Check sheet for the modelled part. Datum: model origin and axes. Units: mm. Give positions to 0.01 mm unless a question says otherwise; leave off trailing zeros. Write each loop counter-clockwise with the first axis right and the second up, starting at its lowest first coordinate (ties: lowest second). Pieces come first, ordered by that corner, then holes. Notation, with made-up numbers: (48, 28.5) -> (101, 28.5) arc R21 cw to (101, 53.5) -> close; hole circle Ø2 at (1, -27). An arc over 180 degrees is marked (long way). Answer as a JSON object with one key per item and string values.
from build123d import *

# Parameters (mm, degrees)
F1_DEPTH = 0.8128
F2_R     = 4.5
F3_DEPTH = 25.4


with BuildPart() as f1:
    # F0 (on Front) → F1 (new body)
    with BuildSketch(Plane.XZ):
        with BuildLine():
            ThreePointArc((-20.832611, 3.624153), (0, 21.1455), (20.832611, 3.624153))
            ThreePointArc((20.832611, 3.624153), (23.001379, -0.147215), (27.08865, -1.637512))
            Line((27.08865, -1.637512), (38.1, -1.637512))
            Line((38.1, -1.637512), (38.1, 33.287488))
            ThreePointArc((38.1, 33.287488), (36.240128, 37.777616), (31.75, 39.637488))
            Line((31.75, 39.637488), (-31.75, 39.637488))
            ThreePointArc((-31.75, 39.637488), (-36.240128, 37.777616), (-38.1, 33.287488))
            Line((-38.1, 33.287488), (-38.1, -1.637512))
            Line((-38.1, -1.637512), (-27.08865, -1.637512))
            ThreePointArc((-27.08865, -1.637512), (-23.001379, -0.147215), (-20.832611, 3.624153))
        make_face()
    extrude(amount=F1_DEPTH)

    # F2 (on face) → F3 (cut)
    with BuildSketch(Plane.XZ.offset(0.8128)):
        with Locations((0, 32.944188)):
            Circle(F2_R)
    extrude(amount=-F3_DEPTH, mode=Mode.SUBTRACT)


solid = f1.part
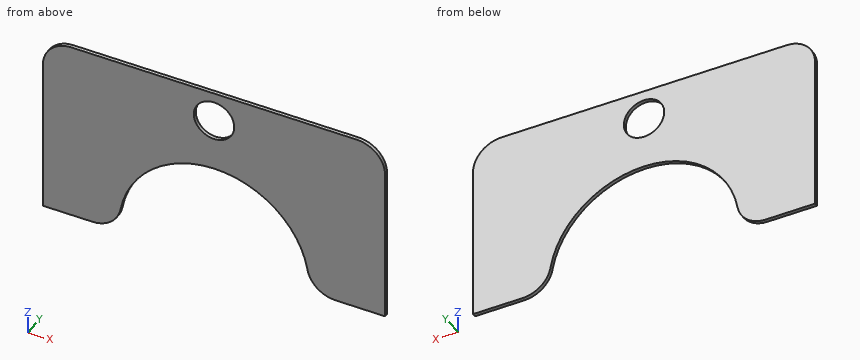
1. Sectioned sample at C-C, the plane y = -0.5. Enter the section's corners in (x, z), plus the area to 3 significant figures.
Determined:
{"outline": "(-38.1, -1.64) -> (-27.09, -1.64) arc R6.35 ccw to (-20.83, 3.62) arc R21.15 cw to (20.83, 3.62) arc R6.35 ccw to (27.09, -1.64) -> (38.1, -1.64) -> (38.1, 33.29) arc R6.35 ccw to (31.75, 39.64) -> (-31.75, 39.64) arc R6.35 ccw to (-38.1, 33.29) -> close; hole circle Ø9 at (0, 32.94)", "area": "2,280 mm^2"}
2. Scan lines: L1, parallel to Z at x = 0, y = -0.15; L2, parallel to X at y = -0.3, z = 31.5; L3, parallel to X at y = -0.3, z = 17. Record each from-to range of solid material in increasing order. Write a range as [from, to].
Determined:
{"L1": "[21.15, 28.44], [37.44, 39.64]", "L2": "[-38.1, -4.26], [4.26, 38.1]", "L3": "[-38.1, -12.58], [12.58, 38.1]"}
3. Sectioned sample at B-B, the plane z = 35.5. Enter the section's corners in (x, y), plus the area to 3 significant figures.
Determined:
{"outline": "(-37.7, -0.81) -> (-3.7, -0.81) -> (-3.7, 0) -> (-37.7, 0) -> close; (3.7, -0.81) -> (37.7, -0.81) -> (37.7, 0) -> (3.7, 0) -> close", "area": "55.3 mm^2"}
4. Go/stop test with a flat-tipped pin: P1, Ø5.5, axis at x = 0, z = 32.94, coming from the +Y side. Record where the tip stops, or that it passes through.
Determined:
{"P1": "through"}
5. Sectioned sample at A-A, the plane x = 0. Enter the section's corners in (y, z).
Determined:
{"outline": "(-0.81, 21.15) -> (0, 21.15) -> (0, 28.44) -> (-0.81, 28.44) -> close; (-0.81, 37.44) -> (0, 37.44) -> (0, 39.64) -> (-0.81, 39.64) -> close"}
